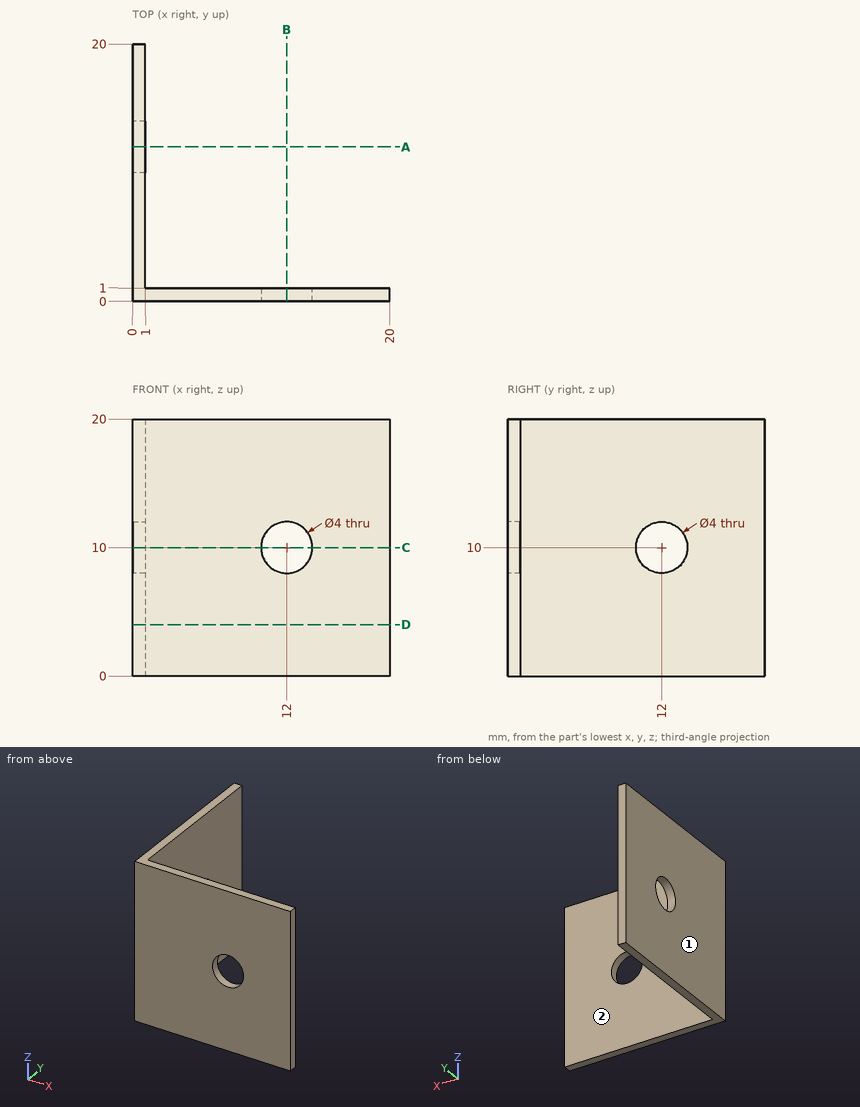
The drawing under review shows one solid part. Ordinate dimensions are in mm from its lowest x, y, z. A direction names the side the tool comes from. Round coordinates to 2 decimals unless told otherwise and drop trailing zeros. Order: outer loops, then holes, each group sorted by start corner. A loop starts at its lowest first (then second) coordinate and runs counter-clockwise, first axis right, second up. Notation, with made-up numbers: (-37, 68) - (2, 68) arc R31 cw to (2, 99) - close; hole circle Ø10 at (23.5, 18). An arc over 180 degrees is marked (long way). Return JSON: item names as keys, results as strings.
Q1. Wall thickness on L1, parallel to Z at x = 12, y = 0.45; L2, parallel to Y at x = 0.3, z = 10; L3, parallel to X at y = 1.25, z = 14: over which ranges is each line inside the solid? List them lowest first. Write a range as [from, to].
Computed values:
{"L1": "z = [0, 8], [12, 20]", "L2": "y = [0, 10], [14, 20]", "L3": "x = [0, 1]"}
Q2. Consider section C-C on z = 10. Write out the cut boundary in (x, y), plus the area to 3 significant figures.
Computed values:
{"outline": "(0, 0) - (10, 0) - (10, 1) - (1, 1) - (1, 10) - (0, 10) - close; (0, 14) - (1, 14) - (1, 20) - (0, 20) - close; (14, 0) - (20, 0) - (20, 1) - (14, 1) - close", "area": "31.0 mm2"}
Q3. Consider section A-A on y = 12. Write out the cut boundary in (x, z).
Computed values:
{"outline": "(0, 0) - (1, 0) - (1, 8) - (0, 8) - close; (0, 12) - (1, 12) - (1, 20) - (0, 20) - close"}
Q4. For pin 1 Ø10 at (x, z) = (2.5, 8) entering from -Y; pin 2 Ø12 at (x, y) = (7.5, 11) entering from -Z; pin 3 Ø5.5 at (x, z) = (6.5, 13.5) entering from +Y, all flat-tipped, find the tip position at first contact; note any pin that passes through.
Computed values:
{"pin 1": "stops at y = 0", "pin 2": "passes through", "pin 3": "stops at y = 1"}
Q5. Machinability: for the marked faces 1 and 2, which of the approach directions +Z, -Z, +X, -X, +Y, -Y give a long, thin tool a straight path to every point of the face, cutting with its end or side? Answer none if there is none.
Computed values:
{"face 1": "+Z, -Z, -X, +Y, -Y", "face 2": "+Z, -Z, +X, +Y"}
Q6. Consider section D-D on z = 4. Write out the cut boundary in (x, y).
Computed values:
{"outline": "(0, 0) - (20, 0) - (20, 1) - (1, 1) - (1, 20) - (0, 20) - close"}
